```python
from build123d import *

# Parameters (mm, degrees)
SKETCH1_W          = 12.71
SKETCH1_H          = 12.7
SKETCH2_R          = 4
CUT_EXTRUDE3_DEPTH = 288.056150001


with BuildPart() as part:
    # Sketch1 → Revolve1 (revolve)
    with BuildSketch(Plane.XY, mode=Mode.PRIVATE) as revolve1_sk:
        with Locations((32.865, 275.296616264)):
            Rectangle(SKETCH1_W, SKETCH1_H)
    revolve(revolve1_sk.sketch.rotate(Axis((0, 0, 0), (0, 1, 0)), 90), axis=Axis((0, 0, 0), (0, 1, 0)))

    # Sketch2 → Cut-Extrude3 (cut, through all)
    with BuildSketch(Plane(origin=(0, 0, 0), x_dir=(1, 0, 0), z_dir=(0, 1, 0))):
        with Locations((-31.176914536, -18)):
            Circle(SKETCH2_R)
        with Locations((36, 0)):
            Circle(SKETCH2_R)
    extrude(amount=CUT_EXTRUDE3_DEPTH, mode=Mode.SUBTRACT)


solid = part.part
```
Could you check a few things on this model? Use its own coordinates, in mm. Round coordinates to 2 decimals unless told otherwise and drop trailing zeros. Loops run counter-clockwise (first coordinate to the right, second up) from the corner with the lowest first, then second, coordinate; pieces in that order, holes last. Notation, with made-up numbers: (33.25, 35.25) - (40.25, 35.25) arc R23 ccw to (40.25, 53.25) - close; hole circle Ø3 at (59.25, 66). An arc over 180 degrees is marked (long way). Answer in a Markdown table with one row per item. Add a question column.
(1) I need wall thicknesses on line 1 along X through (y, z) = (279, 0); line 2 along Z through (x, y) = (36, 275); line 3 along Z through (x, y) = (1.5, 276). Which ranges of each line are inside material? Lowest first, please.
(2) I'm going to push flat-ended pins straight in: pin 1 (1 mm diameter, centred on y = 280.5, z = -4.5, fed in from -X); pin 2 (4 mm diameter, centred on x = -21, z = -9.5, fed in from -Y); pin 3 (3 mm diameter, centred on x = -17.5, y = 276, fed in from +Z); pin 4 (4 mm diameter, centred on x = -12.5, y = 279.5, fed in from +Z). Where does each tip first touch, or does it pass through?
(3) If we section it at D-D (x = 27.5): Please give me the cut outline in (y, z).
(4) If we section it at C-C (y = 274.25): Please give me the cut outline in (x, z).
(5) If we section it at B-B (z = 12): Please give me the cut outline in (x, y), plus the area to 3 significant figures.
(6) If we section it at A-A (x = 0): Please give me the cut outline in (y, z).
(7) If we mould it in two halves opening along X, with no side actions, what happens to faces 1 (the face through (-9.209, 275.386, -38.123)), 2 (the face through (-7.963, 275.386, -25.286)), 3 (the face through (-1, 281.647, -27))? For each: pulls with the +X half, pulls with the -X half, needs draft (parallel to the pull), parting line crosses it, or undercut.
Model answer:
| question | item | result |
|---|---|---|
| 1 | line 1 | x = -39.22 to -26.51, 26.51 to 32 |
| 1 | line 2 | z = -15.56 to -4, 4 to 15.56 |
| 1 | line 3 | z = -39.19 to -26.47, 26.47 to 39.19 |
| 2 | pin 1 | stops at x = -39.02 |
| 2 | pin 2 | passes through |
| 2 | pin 3 | stops at z = 35.81 |
| 2 | pin 4 | stops at z = 37.79 |
| 3 | outline | (268.95, -27.96) - (281.65, -27.96) - (281.65, 27.96) - (268.95, 27.96) - close |
| 4 | outline | (-35.14, 17.43) arc R39.22 ccw (long way) to (39.14, -2.48) arc R4 cw (long way) to (39.14, 2.48) arc R39.22 ccw to (-32.66, 21.71) arc R4 cw (long way) to start; hole circle Ø53.02 at (0, 0) |
| 5 | outline | (-37.34, 268.95) - (-23.64, 268.95) - (-23.64, 281.65) - (-37.34, 281.65) - close; (23.64, 268.95) - (37.34, 268.95) - (37.34, 281.65) - (23.64, 281.65) - close |
| 5 | area | 348 mm² |
| 6 | outline | (268.95, -39.22) - (281.65, -39.22) - (281.65, -26.51) - (268.95, -26.51) - close; (268.95, 26.51) - (281.65, 26.51) - (281.65, 39.22) - (268.95, 39.22) - close |
| 7 | face 1 | parting line crosses it |
| 7 | face 2 | undercut |
| 7 | face 3 | needs draft |
